Read the model definition and answer for the solid it produces. Units are mm, in the model's axes. Face numbers are marked on the shaded views. A direction names the side the tool comes from. Coordinates: 2 decimals unless noted, no trailing zeros. Loops run counter-clockwise (first coordinate to the right, second up) from the corner with the lowest first, then second, coordinate; pieces in that order, holes last. Notation, with made-up numbers: M -11.75,77.5 L 31.25,77.5 A16 cw 31.25,100.5 Z; hole C 33.25,-16 d10. An arc over 180 degrees is marked long. Use one line per item in the form item = value. Start each with the question number.
1. The part is cut by section C-C (z = 3.5). Give the vertices of the cut face in (x, y), plus the area to 3 significant figures.
2. Find the intervals of material crossed by probe 1 along Y at (x, z) = (2.25, 14); probe 2 along Z at (x, y) = (12, 2.75); probe 3 along X at (y, z) = (2.75, 13.75), in increasing order. Write a range as [from, to].
3. Flat-ended cylindrical pins translate along their axes: pin 1 (5 mm diameter, centred on x = -1.5, y = 0.5, fed in from +Z); pin 2 (4 mm diameter, centred on y = -6, z = 20, fed in from -X). Find the tip coordinate at first contact, or state that the pin passes through.
4. For a pull along Y with two mould halves and no side action, classify the marked faces 3, 4 and 5 as released by +Y, released by -Y, zero draft, split by the parting line, or undercut.
5. The part is cut by section A-A (x = 9.5). Give the vertices of the cut face in (y, z).
6. A tool of negligible diameter and unlimited length cuts with its end or side. For the marked faces 1 and 2, from which of +Z, -Z, +X, -X, +Y, -Y can it reach the whole face along a straight path? Write none if from no direction.
7. The part is cut by section B-B (y = 4.75). Give the vertices of the cut face in (x, z), plus the area to 3 significant figures.
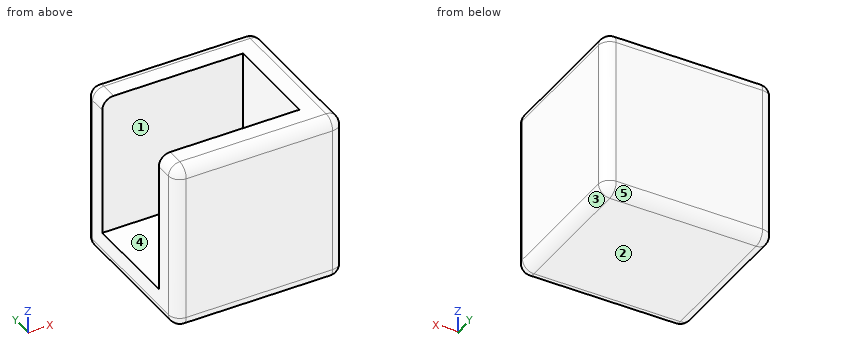
from build123d import *

# Parameters (mm, degrees)
SKETCH_W     = 30
SKETCH_H     = 27.5
PAD_DEPTH    = 5
PAD001_DEPTH = 25
FILLET_R     = 2


with BuildPart() as part:
    # Sketch → Pad (new body)
    with BuildSketch(Plane.XY):
        with Locations((2.5, 0)):
            Rectangle(SKETCH_W, SKETCH_H)
    extrude(amount=-PAD_DEPTH)

    # Sketch001 → Pad001 (join)
    with BuildSketch(Plane.XY):
        Polygon((-12.5, 8.75), (12.5, 8.75), (12.5, -8.75), (-12.5, -8.75), (-12.5, -13.75), (17.5, -13.75), (17.5, 13.75), (-12.5, 13.75), align=None)
    extrude(amount=PAD001_DEPTH)

    # Fillet
    fillet_edges = [part.edges().sort_by_distance(p)[0] for p in [
        (17.5, 0, 25),
        (2.5, -13.75, 25),
        (2.5, 13.75, 25),
        (17.5, 13.75, 10),
        (17.5, -13.75, 10),
        (17.5, 0, -5),
        (2.5, 13.75, -5),
        (-12.5, 13.75, 10),
        (-12.5, 0, -5),
        (-12.5, -13.75, 10),
        (2.5, -13.75, -5),
        (-12.5, -11.25, 25),
        (-12.5, 11.25, 25),
    ]]
    fillet(fillet_edges, radius=FILLET_R)


solid = part.part
Computed values:
q1.outline = M -12.5,-11.75 A2 ccw -10.5,-13.75 L 15.5,-13.75 A2 ccw 17.5,-11.75 L 17.5,11.75 A2 ccw 15.5,13.75 L -10.5,13.75 A2 ccw -12.5,11.75 L -12.5,8.75 L 12.5,8.75 L 12.5,-8.75 L -12.5,-8.75 Z
q1.area = 384 mm²
q2.probe_1 = [-13.75, -8.75], [8.75, 13.75]
q2.probe_2 = [-5, 0]
q2.probe_3 = [12.5, 17.5]
q3.pin_1 = 0
q3.pin_2 = 12.5
q4.face_3 = zero draft
q4.face_4 = undercut
q4.face_5 = released by +Y
q5.outline = M -13.75,-3 A2 ccw -11.75,-5 L 11.75,-5 A2 ccw 13.75,-3 L 13.75,23 A2 ccw 11.75,25 L 8.75,25 L 8.75,0 L -8.75,0 L -8.75,25 L -11.75,25 A2 ccw -13.75,23 Z
q6.face_1 = +Z, -X
q6.face_2 = -Z, +X, -X, +Y, -Y
q7.outline = M -12.5,-3 A2 ccw -10.5,-5 L 15.5,-5 A2 ccw 17.5,-3 L 17.5,23 A2 ccw 15.5,25 L 12.5,25 L 12.5,0 L -12.5,0 Z
q7.area = 272 mm²
